from build123d import *

# Parameters (mm, degrees)
BASEHEAD_DEPTH      = 7.76
SKETCH4_W           = 0.6
SKETCH4_H           = 11.392304845
BOSS_EXTRUDE1_DEPTH = 10


# Read off the part's stored shape, not the designer's step: HeadChamfer
with BuildPart() as part:
    # Sketch1 → BaseHead (new body)
    with BuildSketch(Plane(origin=(0, 0, 0), x_dir=(0, 0, -1), z_dir=(1, 0, 0))):
        Polygon((9, 5.196152423), (9, -5.196152423), (0, -10.392304845), (-9, -5.196152423), (-9, 5.196152423), (0, 10.392304845), align=None)
    extrude(amount=BASEHEAD_DEPTH)

    # HeadChamfer outline → HeadChamfer (revolve, cut)
    with BuildSketch(Plane.YX):
        Polygon((10.392304847, 0.803847578), (9, 0), (10.392304847, 0), align=None)
    revolve(axis=Axis((0, 0, 0), (1, 0, 0)), mode=Mode.SUBTRACT)

    # HeadChamfer 2 outline → HeadChamfer 2 (revolve)
    with BuildSketch(Plane.YX):
        Polygon((6, 7.76), (6, 66.796), (5.036, 67.76), (0, 67.76), (0, 7.76), align=None)
    revolve(axis=Axis((0, 0, 0), (1, 0, 0)))

    # Sketch4 → BearingFace (revolve, cut)
    with BuildSketch(Plane.XY, mode=Mode.PRIVATE) as bearingface_sk:
        with Locations((7.46, 14.696152423)):
            Rectangle(SKETCH4_W, SKETCH4_H)
    revolve(bearingface_sk.sketch.rotate(Axis((0, 0, 0), (1, 0, 0)), 90), axis=Axis((0, 0, 0), (1, 0, 0)), mode=Mode.SUBTRACT)

    # Sketch5 → Boss-Extrude1 (add)
    with BuildSketch(Plane(origin=(62.76, 0, 0), x_dir=(0, 0, -1), z_dir=(1, 0, 0))):
        Polygon((0, 10.392304845), (-9, 5.196152423), (-9, -5.196152423), (0, -10.392304845), (9, -5.196152423), (9, 5.196152423), align=None)
    extrude(amount=-BOSS_EXTRUDE1_DEPTH)


solid = part.part
The listing builds one solid part. Answer for the finished solid, in the listing's coordinates (mm). A direction names the side the tool comes from. Round coordinates to 2 decimals unless told otherwise and drop trailing zeros. Write each loop counter-clockwise with the first axis right and the second up, starting at its lowest first coordinate (ties: lowest second). Pieces come first, ordered by that corner, then holes. Notation, with made-up numbers: M 37.5,39 L 41.5,39 A22 ccw 41.5,61 Z; hole C 61.5,-14 d2. An arc over 180 degrees is marked long. Write each question's results on one line, items separated by ' | '. Start each with the question number.
(1) The part is cut by section A-A, the plane x = 8.5. Write down the section's boundary in (y, z), and give its area (3 significant figures).
(2) Each of these flat-tipped pins is pushed along its axis until it touches: P1, Ø5, axis at x = 24.5, z = -7, coming from the +Y side; P2, Ø4, axis at x = 37, y = -1, coming from the -Z side; P3, Ø2.5, axis at y = -4, z = 7.5, coming from the +X side. Where does it stop, or does it pass through?
(3) For faces 4 (the cylindrical face through (7.464, 8.786, -1.951)), 5 (the flat face through (7.16, 5, -8)), 6 (the flat face through (7.16, -4.5, -8.1)), 7 (the flat face through (7.16, -4.5, 8.1)), determine the directions among +Z, -Z, +X, -X, +Y, -Y from which every point of the face is accessible in a straight line to the end or side of a thin tool.
(4) The part is cut by section B-B, the plane x = 60. Write down the section's boundary in (y, z), and give its area (3 significant figures).
(5) Find the intervals of material crossed by line 1 (X direction, y = -0.5, z = -7.25); line 2 (Z direction, x = 9, y = 3.25); line 3 (Z direction, x = 39.5, y = 5.5), in increasing order.
(6) Determine the mould class of faces 1 (the flat face through (52.76, -2, 6)), 2 (the flat face through (57.83, -7.76, 4.56)), 3 (the conical face through (0.19, -4.65, 8.09)) for opening direction X: +X half, -X half, draft (parallel to the pull), parting line (faces both ways), or undercut.
Worked answers:
1) outline: C 0,0 d12 | area: 113 mm²
2) P1: stops at y = 3.97 | P2: stops at z = -6 | P3: stops at x = 62.76
3) face 4: none | face 5: -Z, +Y | face 6: -Z, -Y | face 7: +Z, -Y
4) outline: M -10.39,0 L -5.2,-9 L 5.2,-9 L 10.39,0 L 5.2,9 L -5.2,9 Z | area: 281 mm²
5) line 1: x = 0 to 7.76, 52.76 to 62.76 | line 2: z = -5.04 to 5.04 | line 3: z = -2.4 to 2.4
6) face 1: undercut | face 2: draft | face 3: -X half
